Geometry check sheet. Reference: drawing and pictorial views, mm from the part's lowest x, y, z. Give positions to 0.01 mm unless a question says otherwise; leave off trailing zeros. Order: outer loops, then holes, each group sorted by start corner. A loop starts at its lowest first (then second) coordinate and runs counter-clockwise, first axis right, second up. Notation, with made-up numbers: (-30, 55.25) -> (29, 55.25) arc R19 ccw to (29, 84.25) -> close; hole circle Ø1 at (47.5, -20). An arc over 180 degrees is marked (long way). Write each question's results on one line, items separated by ' | '. Start each with the question number.
1. Cross-section at A-A, the plane y = 12.75. Enter the section's corners in (x, z).
2. Cross-section at B-B, the plane x = 12.75. Enter the section's corners in (y, z), then the cut area to 3 significant figures.
3. Cross-section at D-D, the plane y = 18.75. Enter the section's corners in (x, z).
4. Material ranges on L1, parallel to Y at x = 12.75, z = 1.7; L2, parallel to Y at x = 12.75, z = 5.4; L3, parallel to X at y = 11.5, z = 1.75, recorded low to high. Write a range as from..to.
5. Cross-section at C-C, the plane z = 3.25. Enter the section's corners in (x, y), then the cut area to 3 significant figures.
6. Mould release check, pull along Y, two halves, no side actions. Record for the marked faces 1, 2 and 3: +Y half, -Y half, draft (parallel to the pull), parting line (faces both ways), or undercut.
7. Depth check by flat-ended pin: pin 1 Ø1.6 at (x, y) = (12.75, 3.05) entering from -Z; pin 2 Ø1.5 at (y, z) = (17.5, 1) entering from +X; pin 3 Ø1 at (x, z) = (18, 5.5) entering from -Y. Enter the tip coordinate at first touch or a pass-through.
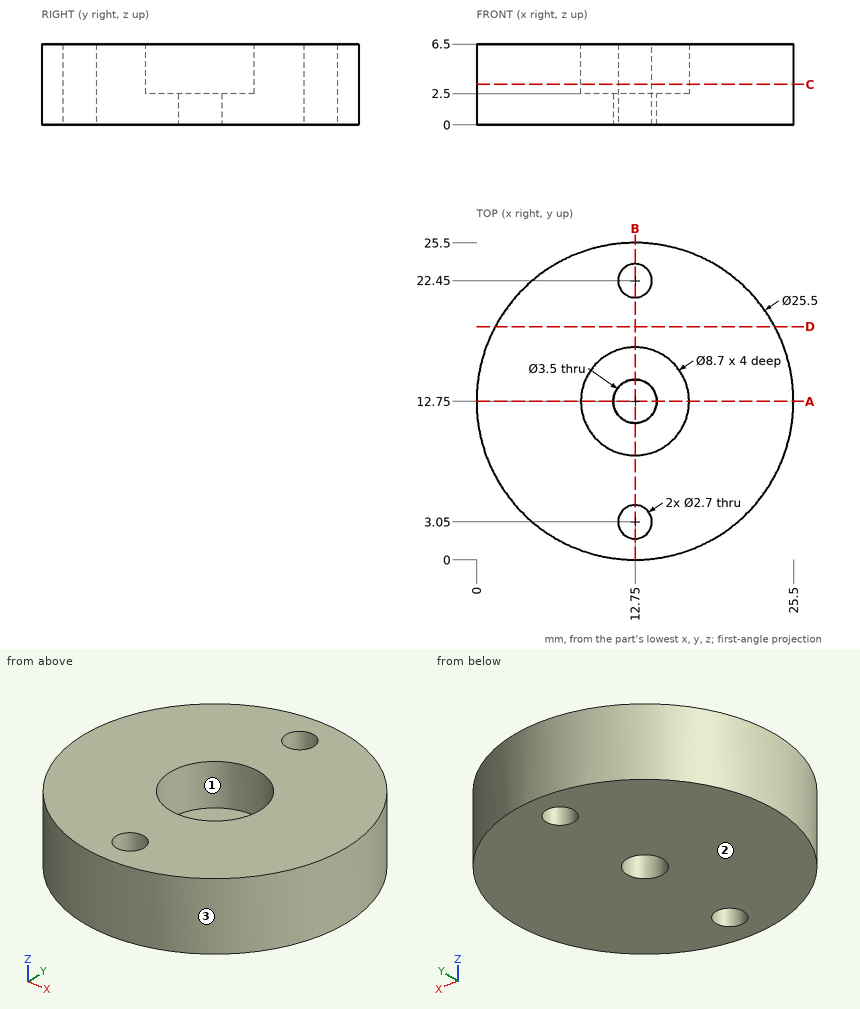
Results below:
1) outline: (0, 0) -> (11, 0) -> (11, 2.5) -> (8.4, 2.5) -> (8.4, 6.5) -> (0, 6.5) -> close; (14.5, 0) -> (25.5, 0) -> (25.5, 6.5) -> (17.1, 6.5) -> (17.1, 2.5) -> (14.5, 2.5) -> close
2) outline: (0, 0) -> (1.7, 0) -> (1.7, 6.5) -> (0, 6.5) -> close; (4.4, 0) -> (11, 0) -> (11, 2.5) -> (8.4, 2.5) -> (8.4, 6.5) -> (4.4, 6.5) -> close; (14.5, 0) -> (21.1, 0) -> (21.1, 6.5) -> (17.1, 6.5) -> (17.1, 2.5) -> (14.5, 2.5) -> close; (23.8, 0) -> (25.5, 0) -> (25.5, 6.5) -> (23.8, 6.5) -> close | area: 87.1 mm²
3) outline: (1.5, 0) -> (24, 0) -> (24, 6.5) -> (1.5, 6.5) -> close
4) L1: y = 0..1.7, 4.4..11, 14.5..21.1, 23.8..25.5 | L2: y = 0..1.7, 4.4..8.4, 17.1..21.1, 23.8..25.5 | L3: x = 0.06..11.53, 13.97..25.44
5) outline: circle Ø25.5 at (12.75, 12.75); hole circle Ø8.7 at (12.75, 12.75); hole circle Ø2.7 at (12.75, 3.05); hole circle Ø2.7 at (12.75, 22.45) | area: 440 mm²
6) face 1: undercut | face 2: draft | face 3: parting line
7) pin 1: passes through | pin 2: stops at x = 24.86 | pin 3: stops at y = 0.92
